CAD build for the part. Positions are in the model's coordinates, mm. A direction names the side the tool comes from. Coordinates: 2 decimals unless noted, no trailing zeros. Loops run counter-clockwise (first coordinate to the right, second up) from the corner with the lowest first, then second, coordinate; pieces in that order, holes last. Notation, with made-up numbers: (83, -18.75) - (100, -18.75) arc R34 ccw to (100, 11.25) - close; hole circle Ø8 at (49, 55). An arc over 180 degrees is marked (long way). Put each result on its own line as item: value.
```python
from build123d import *

# Parameters (mm, degrees)
EXTRUDE_1_DEPTH          = 4
CUT_EXTRUDE_1_REACH      = 162.681
SKETCH_2_R               = 1
CUT_EXTRUDE_2_DEPTH      = 161.68143152
CUT_EXTRUDE_2_DEPTH_BACK = 161.68143152
FILLET_1_R               = 2


with BuildPart() as part:
    # 草图1 → 凸台-拉伸1 (new body)
    with BuildSketch(Plane.XY):
        Polygon((136.299385308, -68.941921014), (136.299385308, -65.041921014), (97.699385308, -65.041921014), (97.699385308, 12.158078986), (136.299385308, 12.158078986), (136.299385308, 16.058078986), (93.799385308, 16.058078986), (93.799385308, -68.941921014), align=None)
    extrude(amount=-EXTRUDE_1_DEPTH)

    # 草图2 → 切除-拉伸1 (cut, up to next)
    with BuildSketch(Plane.XZ.offset(68.941921014), mode=Mode.PRIVATE) as cut_extrude_1_sk1:
        with Locations(Location((134.299385308, -2, 0), (0, 0, 270))):
            Circle(SKETCH_2_R)
    cut_extrude_1_tool1 = extrude(cut_extrude_1_sk1.sketch, amount=-CUT_EXTRUDE_1_REACH, mode=Mode.PRIVATE) & part.part
    cut_extrude_1 = cut_extrude_1_tool1.solids().sort_by_distance((134.299385, -68.941921, -2))[0]
    add(cut_extrude_1, mode=Mode.SUBTRACT)

    # 镜向1: 切除-拉伸1 across plane
    add(cut_extrude_1.mirror(Plane(origin=(0, -26.441921014, 0), x_dir=(0, 0, 1), z_dir=(0, -1, 0))), mode=Mode.SUBTRACT)

    # 草图3 → 切除-拉伸2 (cut, two sides: drawn at the far end of the back side and taken through both)
    with BuildSketch(Plane(origin=(0, 16.058078986, 0), x_dir=(1, 0, 0), z_dir=(0, 1, 0)).offset(-CUT_EXTRUDE_2_DEPTH_BACK)):
        with BuildLine():
            Line((136.299385308, 3.154700538), (136.299385308, 4))
            Line((136.299385308, 4), (134.299385308, 4))
            ThreePointArc((134.299385308, 4), (134.817023399, 3.931851653), (135.299385308, 3.732050808))
            Line((135.299385308, 3.732050808), (136.299385308, 3.154700538))
        make_face()
        with BuildLine():
            Line((135.454085847, 0), (136.031436116, 1))
            ThreePointArc((136.031436116, 1), (136.231236961, 1.48236191), (136.299385308, 2))
            Line((136.299385308, 2), (136.299385308, 1.464101615))
            Line((136.299385308, 1.464101615), (136.299385308, 0))
            Line((136.299385308, 0), (135.454085847, 0))
        make_face()
    extrude(amount=CUT_EXTRUDE_2_DEPTH + CUT_EXTRUDE_2_DEPTH_BACK, mode=Mode.SUBTRACT)

    # 圆角1
    # the kernel refuses this fillet: 2 mm, written as the material it takes off along each edge
    with BuildSketch(Plane(origin=(140.454085847, 16.058078986, 0), x_dir=(0, -1, 0), z_dir=(-1, 0, 0))) as fillet_1_piece_1:
        with BuildLine():
            CenterArc((FILLET_1_R, -FILLET_1_R), FILLET_1_R, 90, 90)
            Line((0, -FILLET_1_R), (0, 0))
            Line((0, 0), (FILLET_1_R, 0))
        make_face()
    extrude(amount=51.654700538, mode=Mode.SUBTRACT)
    with BuildSketch(Plane(origin=(93.799385308, 21.058078986, 0), x_dir=(1, 0, 0), z_dir=(0, -1, 0))) as fillet_1_piece_2:
        with BuildLine():
            CenterArc((FILLET_1_R, -FILLET_1_R), FILLET_1_R, 90, 90)
            Line((0, -FILLET_1_R), (0, 0))
            Line((0, 0), (FILLET_1_R, 0))
        make_face()
    extrude(amount=95, mode=Mode.SUBTRACT)
    with BuildSketch(Plane(origin=(88.799385308, -68.941921014, 0), x_dir=(0, 0, -1), z_dir=(1, 0, 0))) as fillet_1_piece_3:
        with BuildLine():
            CenterArc((FILLET_1_R, FILLET_1_R), FILLET_1_R, 180, 90)
            Line((0, FILLET_1_R), (0, 0))
            Line((0, 0), (FILLET_1_R, 0))
        make_face()
    extrude(amount=51.654700538, mode=Mode.SUBTRACT)


solid = part.part
```
Q1. Pin check, flat tips, straight feed: pin 1 Ø1.2 at (x, z) = (134.3, -2) entering from +Y; pin 2 Ø1 at (x, y) = (98, -5) entering from +Z. Stop position of each tip, or through.
Determined:
pin 1: through
pin 2: z = 0
Q2. Slice it at B-B, the plane y = 1.5. Give the cut face in (x, z), then the cut area to 3 significant figures.
Determined:
outline: (93.8, -4) - (97.7, -4) - (97.7, 0) - (95.8, 0) arc R2 ccw to (93.8, -2) - close
area: 14.7 mm2
Q3. Slice it at A-A, the plane x = 102.5. Give the cut face in (y, z), then the cut area to 3 significant figures.
Determined:
outline: (-68.94, -4) - (-65.04, -4) - (-65.04, 0) - (-66.94, 0) arc R2 ccw to (-68.94, -2) - close; (12.16, -4) - (16.06, -4) - (16.06, -2) arc R2 ccw to (14.06, 0) - (12.16, 0) - close
area: 29.5 mm2
Q4. Tool access for faces 4 (the cylindrical face through (115.347, 15.457, -0.57)), 5 (the flat face through (117, 12.158, -2)): list every direction of +Z, -Z, +X, -X, +Y, -Y with a clear straight run to the whole face (end or side of a thin tool).
Determined:
face 4: +Z, +X, -X, +Y
face 5: +Z, -Z, +X
Q5. Mould opens along X. For faces 1 (the flat face through (97.699, -27, -2)), 2 (the cylindrical face through (94.4, -25.85, -0.57)), 3 (the cylindrical face through (133.916, 14.135, -2.924)) say: +X half, -X half, draft (parallel to the pull), parting line (faces both ways), or undercut.
Determined:
face 1: +X half
face 2: -X half
face 3: undercut
Q6. Wall check: L1, parallel to Y at x = 102.5, z = -2.7; L2, parallel to X at y = 13.8, z = -2; L3, parallel to X at y = -48, z = -3.1. Give the ranges that are in metal, low to high. Write a range as from..to.
Determined:
L1: -68.94..-65.04, 12.16..16.06
L2: 93.8..133.3, 135.3..136.3
L3: 93.8..97.7
